Build history of the part. All positions in model axes, mm. A direction names the side the tool comes from. Coordinates: 2 decimals unless noted, no trailing zeros. Order: outer loops, then holes, each group sorted by start corner. A loop starts at its lowest first (then second) coordinate and runs counter-clockwise, first axis right, second up. Notation, with made-up numbers: (37.25, -10.5) - (70.25, -10.5) arc R11 cw to (70.25, 6.5) - close; hole circle Ø1 at (87.25, -22). An arc over 180 degrees is marked (long way). One line per item, written item: value.
from build123d import *

# Parameters (mm, degrees)
F0_R     = 1.6
F0_R_2   = 12
F1_DEPTH = 3
F2_R     = 1.6
F2_R_2   = 12
F3_DEPTH = 4


with BuildPart() as f1:
    # F0 (on Top) → F1 (new body)
    with BuildSketch(Plane.XY):
        with BuildLine():
            ThreePointArc((50, 33), (47.656854, 38.656854), (42, 41))
            Line((42, 41), (-42, 41))
            ThreePointArc((-42, 41), (-47.656854, 38.656854), (-50, 33))
            Line((-50, 33), (-50, -33))
            ThreePointArc((-50, -33), (-47.656854, -38.656854), (-42, -41))
            Line((-42, -41), (42, -41))
            ThreePointArc((42, -41), (47.656854, -38.656854), (50, -33))
            Line((50, -33), (50, 33))
        make_face()
        with Locations((-15.5, -15.5)):
            Circle(F0_R, mode=Mode.SUBTRACT)
        with BuildLine():
            Line((42, -35), (-42, -35))
            ThreePointArc((-42, -35), (-44, -33), (-42, -31))
            Line((-42, -31), (42, -31))
            ThreePointArc((42, -31), (44, -33), (42, -35))
        make_face(mode=Mode.SUBTRACT)
        with Locations((15.5, -15.5)):
            Circle(F0_R, mode=Mode.SUBTRACT)
        with Locations((-15.5, 15.5)):
            Circle(F0_R, mode=Mode.SUBTRACT)
        Circle(F0_R_2, mode=Mode.SUBTRACT)
        with Locations((15.5, 15.5)):
            Circle(F0_R, mode=Mode.SUBTRACT)
        with BuildLine():
            Line((42, 31), (-42, 31))
            ThreePointArc((-42, 31), (-44, 33), (-42, 35))
            Line((-42, 35), (42, 35))
            ThreePointArc((42, 35), (44, 33), (42, 31))
        make_face(mode=Mode.SUBTRACT)
    extrude(amount=F1_DEPTH)

    # F2 (on face) → F3 (join)
    with BuildSketch(Plane.XY.offset(3)):
        with BuildLine():
            ThreePointArc((21, 17), (19.828427, 19.828427), (17, 21))
            Line((17, 21), (-17, 21))
            ThreePointArc((-17, 21), (-19.828427, 19.828427), (-21, 17))
            Line((-21, 17), (-21, -17))
            ThreePointArc((-21, -17), (-19.828427, -19.828427), (-17, -21))
            Line((-17, -21), (17, -21))
            ThreePointArc((17, -21), (19.828427, -19.828427), (21, -17))
            Line((21, -17), (21, 17))
        make_face()
        with Locations((-15.5, -15.5)):
            Circle(F2_R, mode=Mode.SUBTRACT)
        with Locations((15.5, -15.5)):
            Circle(F2_R, mode=Mode.SUBTRACT)
        with Locations((-15.5, 15.5)):
            Circle(F2_R, mode=Mode.SUBTRACT)
        Circle(F2_R_2, mode=Mode.SUBTRACT)
        with Locations((15.5, 15.5)):
            Circle(F2_R, mode=Mode.SUBTRACT)
    extrude(amount=F3_DEPTH)


solid = f1.part
1. Band-saw the part on C-C, the plane x = -37. Give the cut face in (y, z), and give its area (3 significant figures).
Values found:
outline: (-41, 0) - (-35, 0) - (-35, 3) - (-41, 3) - close; (-31, 0) - (31, 0) - (31, 3) - (-31, 3) - close; (35, 0) - (41, 0) - (41, 3) - (35, 3) - close
area: 222 mm2
2. Band-saw the part on B-B, the plane x = 0. Give the cut face in (y, z).
Values found:
outline: (-41, 0) - (-35, 0) - (-35, 3) - (-41, 3) - close; (-31, 0) - (-12, 0) - (-12, 7) - (-21, 7) - (-21, 3) - (-31, 3) - close; (12, 0) - (31, 0) - (31, 3) - (21, 3) - (21, 7) - (12, 7) - close; (35, 0) - (41, 0) - (41, 3) - (35, 3) - close
3. 3-axis set-ups, long thin cutter, end or side, ignore diameter. For faces 1 (the face through (-1, 35, 1)), 2 (the face through (19.797, -19.859, 4.972)), 3 (the face through (-19.859, -19.797, 4.972)): which of +Z, -Z, +X, -X, +Y, -Y reach the whole face in a straight line?
Values found:
face 1: +Z, -Z
face 2: +Z, +X, -Y
face 3: +Z, -X, -Y
4. Flat gauge pins, fed straight in: P1, Ø3, axis at y = -2, z = 5.5, coming from the +X side; P2, Ø2, axis at x = 33.5, y = -29.5, coming from the +Z side; P3, Ø2, axis at y = 2, z = 5.5, coming from the -X side; P4, Ø1.9, axis at x = 15.5, y = 15.5, coming from the +Z side. Where does each tip first touch, or does it go through?
Values found:
P1: stops at x = 21
P2: stops at z = 3
P3: stops at x = -21
P4: passes through
5. Band-saw the part on A-A, the plane y = 15.5. Give the cut face in (x, z), and give its area (3 significant figures).
Values found:
outline: (-50, 0) - (-17.1, 0) - (-17.1, 7) - (-21, 7) - (-21, 3) - (-50, 3) - close; (-13.9, 0) - (13.9, 0) - (13.9, 7) - (-13.9, 7) - close; (17.1, 0) - (50, 0) - (50, 3) - (21, 3) - (21, 7) - (17.1, 7) - close
area: 423 mm2
6. Band-saw the part on D-D, the plane y = 0. Give the cut face in (x, z), and give its area (3 significant figures).
Values found:
outline: (-50, 0) - (-12, 0) - (-12, 7) - (-21, 7) - (-21, 3) - (-50, 3) - close; (12, 0) - (50, 0) - (50, 3) - (21, 3) - (21, 7) - (12, 7) - close
area: 300 mm2
7. Probe line 1 along Y through (x, z) = (-15.5, 5.25); line 2 along Y through (x, z) = (-43.5, 1.75); line 3 along Y through (x, z) = (-11, 1.5). List the from-to ranges inside material, lowest first.
Values found:
line 1: y = -21 to -17.1, -13.9 to 13.9, 17.1 to 21
line 2: y = -40.86 to -34.32, -31.68 to 31.68, 34.32 to 40.86
line 3: y = -41 to -35, -31 to -4.8, 4.8 to 31, 35 to 41
8. Two-plate mould, pull along X, no slides. Class faces 4 (the face through (1, 41, 1)), 5 (the face through (-21, 0, 5)), 6 (the face through (44, -33, 1)): pulls with the +X half, pulls with the -X half, needs draft (parallel to the pull), parting line crosses it, or undercut.
Values found:
face 4: needs draft
face 5: pulls with the -X half
face 6: undercut
